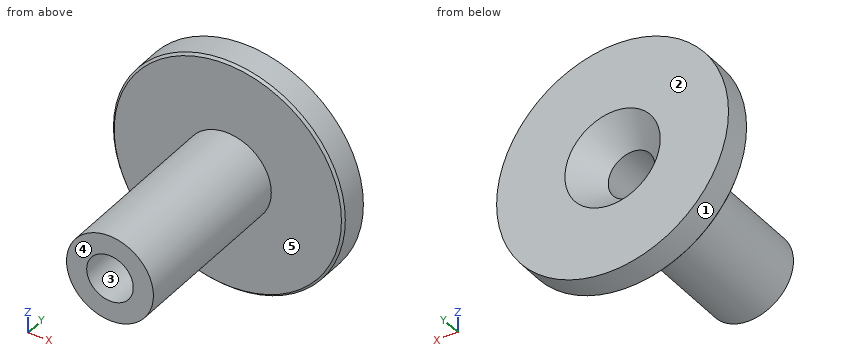
from build123d import *

# Parameters (mm, degrees)
CSK_FOR_10_FLAT_HEAD_SOCKET_CAP_SCREW1_D           = 5.1054
CSK_FOR_10_FLAT_HEAD_SOCKET_CAP_SCREW1_CSINK_D     = 10.4394
CSK_FOR_10_FLAT_HEAD_SOCKET_CAP_SCREW1_CSINK_ANGLE = 82
CHAMFER1_SIZE                                      = 0.254


with BuildPart() as part:
    # Sketch2 → Revolve1 (revolve)
    with BuildSketch(Plane.XY, mode=Mode.PRIVATE) as revolve1_sk:
        Polygon((0, 10.140493615), (-12.7, 10.140493615), (-12.7, 6.965493615), (-4.7625, 6.965493615), (-4.7625, -12.084506385), (0, -12.084506385), align=None)
    revolve(revolve1_sk.sketch.rotate(Axis((0, -12.084506385, 0), (0, 1, 0)), 180), axis=Axis((0, -12.084506385, 0), (0, 1, 0)))

    # CSK for #10 Flat Head Socket Cap Screw1 (through all)
    with Locations(Plane(origin=(0, 10.140493615, 0), x_dir=(1, 0, 0), z_dir=(0, 1, 0))):
        with Locations((0, 0)):
            CounterSinkHole(CSK_FOR_10_FLAT_HEAD_SOCKET_CAP_SCREW1_D / 2, CSK_FOR_10_FLAT_HEAD_SOCKET_CAP_SCREW1_CSINK_D / 2, counter_sink_angle=CSK_FOR_10_FLAT_HEAD_SOCKET_CAP_SCREW1_CSINK_ANGLE)

    # Chamfer1
    chamfer1_edges = [part.edges().sort_by_distance(p)[0] for p in [
        (-12.7, 6.965493615, 0),
    ]]
    chamfer(chamfer1_edges, length=CHAMFER1_SIZE)


solid = part.part
Read the model definition and answer for the solid it produces. Units are mm, in the model's axes. Face numbers are marked on the shaded views. A direction names the side the tool comes from. Coordinates: 2 decimals unless noted, no trailing zeros. Order: outer loops, then holes, each group sorted by start corner. A loop starts at its lowest first (then second) coordinate and runs counter-clockwise, first axis right, second up. Notation, with made-up numbers: M 23.25,-10 L 35.25,-10 A20 cw 35.25,-1 Z; hole C -18.5,-19 d3. An arc over 180 degrees is marked long. Put each result on its own line as item: value. Start each with the question number.
Item 1: Section A-A, the plane x = 0 is taken. Determine the outline of the cut face in (y, z), plus the area to 3 significant figures.
Item 2: The mould has two halves that part along X. Classify the marked faces 1, 2 and 3: +X half, -X half, draft (parallel to the pull), parting line (faces both ways), or undercut.
Item 3: Section B-B, the plane z = 0 is taken. Determine the outline of the cut face in (x, y), plus the area to 3 significant figures.
Item 4: Section C-C, the plane y = -1.25 is taken. Determine the outline of the cut face in (x, z) (1 decimal).
Item 5: Consider probe 1 along Z at (x, y) = (0, -2.25); probe 2 along Y at (x, z) = (3, -6.5); probe 3 along X at (y, z) = (-6.5, -1). Determine where each line is inside the solid, lowest interval first. Write a range as [from, to].
Item 6: Given pin 1 Ø10 at (y, z) = (-5.5, -4) entering from -X; pin 2 Ø8 at (x, y) = (4, -7) entering from -Z; pin 3 Ø10 at (y, z) = (4.5, 5) entering from -X, each flat-ended and moving along its own axis, determine where each tip first touches the part or whether it passes through.
Item 7: For the marked faces 4 and 5, determine the directions among +Z, -Z, +X, -X, +Y, -Y from which every point of the face is accessible in a straight line to the end or side of a thin tool.
Computed:
1. outline: M -12.08,-4.76 L 6.97,-4.76 L 6.97,-12.45 L 7.22,-12.7 L 10.14,-12.7 L 10.14,-5.22 L 7.07,-2.55 L -12.08,-2.55 Z; M -12.08,2.55 L 7.07,2.55 L 10.14,5.22 L 10.14,12.7 L 7.22,12.7 L 6.97,12.45 L 6.97,4.76 L -12.08,4.76 Z
1. area: 140 mm2
2. face 1: parting line
2. face 2: draft
2. face 3: undercut
3. outline: M -12.7,7.22 L -12.45,6.97 L -4.76,6.97 L -4.76,-12.08 L -2.55,-12.08 L -2.55,7.07 L -5.22,10.14 L -12.7,10.14 Z; M 2.55,-12.08 L 4.76,-12.08 L 4.76,6.97 L 12.45,6.97 L 12.7,7.22 L 12.7,10.14 L 5.22,10.14 L 2.55,7.07 Z
3. area: 140 mm2
4. outline: C 0,0 d9.5; hole C 0,0 d5.1
5. probe 1: z = [-4.76, -2.55], [2.55, 4.76]
5. probe 2: y = [6.97, 10.14]
5. probe 3: x = [-4.66, -2.35], [2.35, 4.66]
6. pin 1: stops at x = -4.76
6. pin 2: stops at z = -4.76
6. pin 3: stops at x = -12.67
7. face 4: +Z, -Z, +X, -X, -Y
7. face 5: -Y
